Build history of the part. All positions in model axes, mm. A direction names the side the tool comes from. Give positions to 0.01 mm unless a question says otherwise; leave off trailing zeros. Write each loop counter-clockwise with the first axis right and the second up, starting at its lowest first coordinate (ties: lowest second). Pieces come first, ordered by that corner, then holes. Notation, with made-up numbers: (66, 49.5) -> (89, 49.5) arc R21 cw to (89, 78.5) -> close; hole circle Ø2 at (18.25, 84). An arc over 180 degrees is marked (long way). One line per question, with ' | ' between items. Start each with the question number.
(1) Band-saw the part on D-D, the plane y = -14.5. Give the cut face in (x, z), and give its area (3 significant figures).
(2) Tool access for faces 4 (the flat face through (-33, -1.5, -20)), 5 (the cylindrical face through (32.53, -1.13, -23.5)), 6 (the flat face through (76, -1, -54.926)): list every direction of +Z, -Z, +X, -X, +Y, -Y with a clear straight run to the whole face (end or side of a thin tool).
(3) Band-saw the part on C-C, the plane x = 19. Give the cut face in (y, z), and give its area (3 significant figures).
(4) Pin check, flat tips, straight feed: P1, Ø8, axis at x = 35, y = 6.5, coming from the +Z side; P2, Ø5, axis at y = -6.5, z = -43, coming from the -X side; P3, Ø1.5, axis at x = -43, z = -24.5, coming from the -Y side. Stop position of each tip, or through.
(5) Pull direction X, two halves, no side cores. Call faces 1 (the flat face through (77.25, -1, -19)), 2 (the flat face through (-33, 1.5, -20)), 3 (the cylindrical face through (-57.73, 0.02, -20.98)): released by +X, released by -X, zero draft, split by the parting line, or undercut.
(6) Band-saw the part on A-A, the plane z = -34.5. Give the cut face in (x, y).
(7) Band-saw the part on B-B, the plane y = 0. Give the cut face in (x, z), and give its area (3 significant figures).
(8) Drill centre lines: probe 1 along Y at (x, z) = (-19, -22); probe 2 along X at (y, z) = (-14.25, -44.5); probe 3 along X at (y, z) = (0, -41). Where is each one in solid material? Low to high. Write a range as from..to.
Autodesk Inventor part; units mm, degrees
ref_plane "YZ Plane" through (0, 0, 0) normal (1, 0, 0) x (0, 1, 0)
ref_plane "XZ Plane" through (0, 0, 0) normal (0, 1, 0) x (-1, 0, 0)
ref_plane "XY Plane" through (0, 0, 0) normal (0, 0, 1) x (1, 0, 0)
sketch "Skizze1" plane through (0, 0, 0) normal (0, 1, 0) x (-1, 0, 0)
  circle A0 centre (32.7504, -19.9257) radius 25
  line L0 (32.7504, -19.9257) -> (-77.2496, -19.9257)
  line L1 (-77.2496, -19.9257) -> (-77.2496, -23.6757)
  line L2 (-77.2496, -23.6757) -> (8.0333, -23.6757)
  line L3 (8.0333, -23.6757) -> (8.0333, -19.9257)
  point P0 (0, 0)
  dimension "d4" = 50
  dimension "d9" = 110
  dimension "d10" = 3.75
extrude "Extrusion1" add sketch "Skizze1" along normal blind 1.5 and the other way blind 1.5 contours L3 L0 A0 | A0 L0 L3
revolve "Umdrehung1" add sketch "Skizze1" angle 360 about axis through (-32.7504, 0, -19.9257) along (1, 0, 0) picked at (7.9809, -22.0108) contours L2 L1 L0 A0 | A0 L0 L3
sketch "Skizze2" plane through (77.2496, 0, -19.9257) normal (1, 0, 0) x (0, 0, -1)
  line L0 (35, -16.5) -> (-35, -16.5)
  line L1 (-35, -16.5) -> (-35, 13.5)
  line L2 (-35, 13.5) -> (35, 13.5)
  line L3 (35, 13.5) -> (35, -16.5)
  line L4 (-25, -1.5) -> (25, -1.5)
  line L5 (35, -16.5) -> (-35, 13.5) construction
  line L6 (-35, -16.5) -> (35, 13.5) construction
  point P0 (-19.9257, 0)
  point P1 (0, -1.5)
  point P2 (-3.75, 0)
  point P3 (3.75, 0)
  dimension "d14" = 70
  dimension "d15" = 30
extrude "Extrusion2" add sketch "Skizze2" against normal blind 3
properties part number "Kreisverkehrsschild"
Results:
1) outline: (74.25, -54.93) -> (77.25, -54.93) -> (77.25, 15.07) -> (74.25, 15.07) -> close | area: 210 mm²
2) face 4: +Z, -Z, -X, -Y | face 5: none | face 6: -Z, +X, -X, +Y, -Y
3) outline: circle Ø7.5 at (0, -19.93) | area: 44.2 mm²
4) P1: stops at z = -17.13 | P2: stops at x = 74.25 | P3: stops at y = -1.5
5) face 1: released by +X | face 2: zero draft | face 3: undercut
6) outline: (-53.06, -1.5) -> (-12.44, -1.5) -> (-12.44, 1.5) -> (-53.06, 1.5) -> close; (74.25, -16.5) -> (77.25, -16.5) -> (77.25, 13.5) -> (74.25, 13.5) -> close
7) outline: (-8.03, -23.68) -> (74.25, -23.68) -> (74.25, -54.93) -> (77.25, -54.93) -> (77.25, 15.07) -> (74.25, 15.07) -> (74.25, -16.18) -> (-8.03, -16.18) arc R25 ccw (long way) to start | area: 2,790 mm²
8) probe 1: y = -1.5..1.5 | probe 2: x = 74.25..77.25 | probe 3: x = -46.2..-19.3, 74.25..77.25
